```python
from build123d import *

# Parameters (mm, degrees)
F1_DEPTH = 12.5
F2_R     = 2.3120560343
F3_DEPTH = 26.251
F4_R     = 5
F5_R     = 1


with BuildPart() as f1:
    # F0 (on Right) → F1 (new body, symmetric)
    with BuildSketch(Plane.YZ):
        with BuildLine():
            ThreePointArc((1, 16.2192015833), (16.25, 0), (1, -16.2192015833))
            Line((1, -16.2192015833), (1, -39.2372590786))
            ThreePointArc((1, -39.2372590786), (4.0118599408, -39.0444295619), (7, -38.6207521936))
            Line((7, -38.6207521936), (7, -28.1777318701))
            ThreePointArc((7, -28.1777318701), (7.6968075003, -25.9224938479), (9.5443367466, -24.453387006))
            ThreePointArc((9.5443367466, -24.453387006), (26.25, 0), (9.5443367466, 24.453387006))
            ThreePointArc((9.5443367466, 24.453387006), (7.6968075003, 25.9224938479), (7, 28.1777318701))
            Line((7, 28.1777318701), (7, 38.6207521936))
            ThreePointArc((7, 38.6207521936), (4.0118599408, 39.0444295619), (1, 39.2372590786))
            Line((1, 39.2372590786), (1, 16.2192015833))
        make_face()
    extrude(amount=F1_DEPTH, both=True)

    # F2 (on Front) → F3 (cut, through all)
    with BuildSketch(Plane.XZ):
        with Locations((6.896616891, 32.556977123)):
            Circle(F2_R)
        with Locations((-6.896616891, 32.556977123)):
            Circle(F2_R)
        with Locations((-6.896616891, -32.556977123)):
            Circle(F2_R)
        with Locations((6.896616891, -32.556977123)):
            Circle(F2_R)
    extrude(amount=-F3_DEPTH, mode=Mode.SUBTRACT)

    # F4
    f4_edges = [f1.edges().sort_by_distance(p)[0] for p in [
        (12.5, 4.01186, 39.04443),
        (-12.5, 4.01186, 39.04443),
        (12.5, 4.01186, -39.04443),
        (-12.5, 4.01186, -39.04443),
    ]]
    fillet(f4_edges, radius=F4_R)

    # F5
    f5_edges = [f1.edges().sort_by_distance(p)[0] for p in [
        (-12.5, 1, -25.2273),
        (-12.5, 4.01565, -34.013777),
        (-12.5, 16.25, 0),
        (-12.5, 7, -30.852387),
        (-12.5, 1, 25.2273),
        (-12.5, 7.696808, -25.922494),
        (-12.5, 4.01565, 34.013777),
        (-12.5, 26.25, 0),
        (-12.5, 7, 30.852387),
        (-12.5, 7.696808, 25.922494),
        (12.5, 1, -25.2273),
        (12.5, 4.01565, -34.013777),
        (12.5, 16.25, 0),
        (12.5, 7, -30.852387),
        (12.5, 1, 25.2273),
        (12.5, 7.696808, -25.922494),
        (12.5, 4.01565, 34.013777),
        (12.5, 26.25, 0),
        (12.5, 7, 30.852387),
        (12.5, 7.696808, 25.922494),
    ]]
    fillet(f5_edges, radius=F5_R)


solid = f1.part
```
The listing builds one solid part. Answer for the finished solid, in the listing's coordinates (mm). A direction names the side the tool comes from. Coordinates: 2 decimals unless noted, no trailing zeros. Loops run counter-clockwise (first coordinate to the right, second up) from the corner with the lowest first, then second, coordinate; pieces in that order, holes last. Notation, with made-up numbers: (-15.5, 71.25) - (30.5, 71.25) arc R7 cw to (30.5, 83.25) - close; hole circle Ø4 at (-9.5, 57.5). An arc over 180 degrees is marked (long way). Use a Markdown table: item, result. Add a question column.
1) Find the intervals of material crossed by line 1 (Z direction, x = -7.5, y = 4.5); line 2 (Z direction, x = -9, y = 4.25); line 3 (Z direction, x = -2.75, y = 6.5), in increasing order.
2) The part is cut by section B-B, the plane x = -8.25. State how many separate pieces and enclosed holes the cut face has, and give its area (3 significant figures).
3) The part is cut by section A-A, the plane z = 0. Give the vertices of the cut face in (x, y).
4) The mould has two halves that part along X. Classify faces 1 (the cylindrical face through (-8.601, 3.958, -30.994)), 2 (the flat face through (-12.5, 19, 0)), 3 (the cylindrical face through (0.161, 26.246, -0.44)): released by +X, released by -X, zero draft, split by the parting line, or undercut.
5) For faces 4 (the flat face through (0, 7, 33)), 5 (the flat face through (0, 7, -33)), 6 (the cylindrical face through (6.6, 3.96, 34.85)), determine the directions among +Z, -Z, +X, -X, +Y, -Y from which every point of the face is accessible in a straight line to the end or side of a thin tool.
6) Given pin 1 (1 mm diameter, centred on x = -9.5, z = 8.5, fed in from -Y); pin 2 (10.5 mm diameter, centred on x = -1, z = -34, fed in from +Y); pin 3 (5 mm diameter, centred on x = 4, z = -16.5, fed in from +Y) (3 decimals); pin 4 (4 mm diameter, centred on y = 9.5, z = 8.5, fed in from -X), each flat-ended and moving along its own axis, determine where each tip first touches the part or whether it passes through.
Here are the results:
| question | item | result |
|---|---|---|
| 1 | line 1 | z = -38.99 to -34.79, -30.33 to -15.61, 15.61 to 30.33, 34.79 to 38.99 |
| 1 | line 2 | z = -38.79 to -33.52, -31.6 to -15.68, 15.68 to 31.6, 33.52 to 38.79 |
| 1 | line 3 | z = -38.64 to -14.89, 14.89 to 38.64 |
| 2 | separate pieces | 3 |
| 2 | enclosed holes | 0 |
| 2 | area | 762 mm^2 |
| 3 | outline | (-12.5, 17.25) arc R1 ccw to (-11.5, 16.25) - (11.5, 16.25) arc R1 ccw to (12.5, 17.25) - (12.5, 25.25) arc R1 ccw to (11.5, 26.25) - (-11.5, 26.25) arc R1 ccw to (-12.5, 25.25) - close |
| 4 | face 1 | undercut |
| 4 | face 2 | released by -X |
| 4 | face 3 | zero draft |
| 5 | face 4 | +Z, +X, -X, +Y |
| 5 | face 5 | -Z, +X, -X, +Y |
| 5 | face 6 | +Y, -Y |
| 6 | pin 1 | stops at y = 13.53 |
| 6 | pin 2 | stops at y = 7 |
| 6 | pin 3 | stops at y = 22.205 |
| 6 | pin 4 | passes through |
